Autodesk Inventor part; units mm, degrees
ref_plane "YZ Plane" through (0, 0, 0) normal (1, 0, 0) x (0, 1, 0)
ref_plane "XZ Plane" through (0, 0, 0) normal (0, 1, 0) x (-1, 0, 0)
ref_plane "XY Plane" through (0, 0, 0) normal (0, 0, 1) x (1, 0, 0)
sketch "Эскиз1" plane through (0, 0, 0) normal (0, 1, 0) x (-1, 0, 0)
  line L0 (0, 0) -> (80, 0)
  line L1 (80, 0) -> (80, -100)
  line L2 (80, -100) -> (0, -100)
  line L3 (0, -100) -> (0, 0)
  dimension "d0" = 80
  dimension "d1" = 100
extrude "Выдавливание1" add sketch "Эскиз1" along normal blind 1.5
sketch "Эскиз2" plane through (0, 1.5, 0) normal (0, 1, 0) x (1, 0, 0)
  circle A0 centre (-4.5, 94) radius 1.25
  circle A1 centre (-4.5, 6) radius 1.25
  circle A2 centre (-75.5, 6) radius 1.25
  line L0 (0, 0) -> (0, 100)
  line L1 (0, 100) -> (-80, 100)
  line L2 (-80, 0) -> (0, 0)
  line L3 (-80, 100) -> (-80, 0)
  dimension "d4" = 2.5
  dimension "d5" = 2.5
  dimension "d6" = 2.5
  dimension "d7" = 4.5
  dimension "d8" = 6
  dimension "d9" = 4.5
  dimension "d10" = 6
  dimension "d11" = 4.5
  dimension "d12" = 6
sketch "Эскиз3" plane through (0, 1.5, 0) normal (0, 1, 0) x (1, 0, 0)
  line L0 (-80, 0) -> (0, 0)
  line L1 (0, 0) -> (-9, 0)
  line L2 (-9, 0) -> (-9, 12)
  line L3 (-9, 12) -> (0, 12)
  line L4 (0, 12) -> (0, 0)
  line L5 (0, 100) -> (-80, 100)
  line L6 (0, 100) -> (-9, 100)
  line L7 (-9, 100) -> (-9, 88)
  line L8 (-9, 88) -> (0, 88)
  line L9 (0, 88) -> (0, 100)
  line L10 (-80, 100) -> (-80, 0)
  line L11 (-80, 0) -> (-71, 0)
  line L12 (-71, 0) -> (-71, 12)
  line L13 (-71, 12) -> (-80, 12)
  line L14 (-80, 12) -> (-80, 0)
  dimension "d13" = 9
  dimension "d14" = 12
  dimension "d15" = 9
  dimension "d16" = 12
  dimension "d17" = 9
  dimension "d18" = 12
extrude "Выдавливание2" add sketch "Эскиз3" along normal blind 5
extrude "Выдавливание3" cut sketch "Эскиз2" along normal blind 5 contours A0 | A1 | A2
fillet "Сопряжение1" radius 2 3 edges at (0, 3.25, 0) (0, 3.25, -100) (-80, 3.25, 0)
properties part number "FLC_Holder"
Could you check a few things on this model? Use its own coordinates, in mm. A direction names the side the tool comes from. Give positions to 0.01 mm unless a question says otherwise; leave off trailing zeros. Order: outer loops, then holes, each group sorted by start corner. A loop starts at its lowest first (then second) coordinate and runs counter-clockwise, first axis right, second up.
Q1. Suppose I cut it at C-C, the plane z = -94. Write out the boundary of the cut face in (x, y).
Q2. Suppose I cut it at D-D, the plane z = -6. Write out the boundary of the cut face in (x, y), and give its area (3 significant figures).
Q3. If I drill on line 1 along X through (y, z) = (2.5, -6); line 2 along Z through (x, y) = (-4.5, 5.1); line 3 along X through (y, z) = (3.25, -8), over which ranges is the centre line in solid material (lowest first)?
Q4. For faces 1 (the flat face through (-9, 4, -94)), 2 (the cylindrical face through (-4.77, 3.96, -7.22)), 3 (the flat face through (-75, 4, -12)), 4 (the flat face through (-71, 4, -6)), 5 (the flat face through (-5, 4, -12)), which set-ups out of +Z, -Z, +X, -X, +Y, -Y let a thin tool reach every point of the face, with its end or its side?
Q5. Suppose I cut it at A-A, the plane y = 5.5. Write out the boundary of the cut face in (x, z), and give its area (3 significant figures).
Q6. Suppose I cut it at B-B, the plane x = -4.5. Write out the boundary of the cut face in (y, z).
Q7. We'd pull the mould along X, two halves only. Please class faces 6 (the flat face through (-5, 4, -88)), 7 (the cylindrical face through (-4.66, 3.96, -92.76)), 8 (the flat face through (-76, 1.5, -6)), 9 (the cylindrical face through (-0.6, 3.3, -0.57)): +X half, -X half, draft (parallel to the pull), parting line (faces both ways), or undercut.
Q8. I'm going to push flat-ended pins straight in: P1, Ø2, axis at x = -75.5, z = -6, coming from the +Y side; P2, Ø1, axis at x = -14, y = 2.5, coming from the +Z side; P3, Ø2.5, axis at x = -73.5, y = 3.5, coming from the -Z side. Where does each tip first touch, or does it pass through?
Solution:
1. outline: (-80, 0) - (0, 0) - (0, 6.5) - (-3.25, 6.5) - (-3.25, 1.5) - (-5.75, 1.5) - (-5.75, 6.5) - (-9, 6.5) - (-9, 1.5) - (-80, 1.5) - close
2. outline: (-80, 0) - (0, 0) - (0, 6.5) - (-3.25, 6.5) - (-3.25, 1.5) - (-5.75, 1.5) - (-5.75, 6.5) - (-9, 6.5) - (-9, 1.5) - (-71, 1.5) - (-71, 6.5) - (-74.25, 6.5) - (-74.25, 1.5) - (-76.75, 1.5) - (-76.75, 6.5) - (-80, 6.5) - close
2. area: 185 mm2
3. line 1: x = -80 to -76.75, -74.25 to -71, -9 to -5.75, -3.25 to 0
3. line 2: z = -100 to -95.25, -92.75 to -88, -12 to -7.25, -4.75 to 0
3. line 3: x = -80 to -71, -9 to 0
4. face 1: +Z, -Z, -X, +Y
4. face 2: +Y
4. face 3: -Z, +X, -X, +Y
4. face 4: +Z, -Z, +Y
4. face 5: +X, -X, +Y
5. outline: (-80, -12) - (-71, -12) - (-71, 0) - (-78, 0) arc R2 ccw to (-80, -2) - close; (-9, -100) - (-2, -100) arc R2 ccw to (0, -98) - (0, -88) - (-9, -88) - close; (-9, -12) - (0, -12) - (0, -2) arc R2 ccw to (-2, 0) - (-9, 0) - close; hole circle Ø2.5 at (-75.5, -6); hole circle Ø2.5 at (-4.5, -94); hole circle Ø2.5 at (-4.5, -6)
5. area: 307 mm2
6. outline: (0, -100) - (6.5, -100) - (6.5, -95.25) - (1.5, -95.25) - (1.5, -92.75) - (6.5, -92.75) - (6.5, -88) - (1.5, -88) - (1.5, -12) - (6.5, -12) - (6.5, -7.25) - (1.5, -7.25) - (1.5, -4.75) - (6.5, -4.75) - (6.5, 0) - (0, 0) - close
7. face 6: draft
7. face 7: undercut
7. face 8: undercut
7. face 9: +X half
8. P1: stops at y = 1.5
8. P2: passes through
8. P3: stops at z = -12
